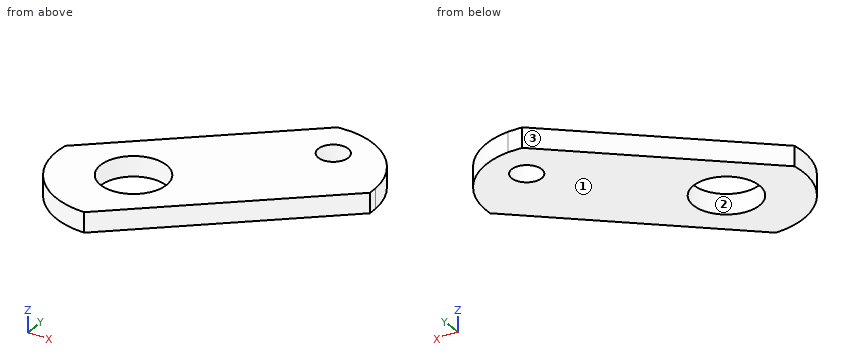
```python
from build123d import *

# Parameters (mm, degrees)
SKETCH1_W           = 38.1
SKETCH1_H           = 30.48
BOSS_EXTRUDE1_DEPTH = 2.54
SKETCH2_R           = 1.905
SKETCH2_R_2         = 4.191
CUT_EXTRUDE1_DEPTH  = 49.857875517
CUT_EXTRUDE3_DEPTH  = 2.54
CUT_EXTRUDE4_DEPTH  = 2.54
CUT_EXTRUDE5_DEPTH  = 2.54


with BuildPart() as part:
    # Sketch1 → Boss-Extrude1 (new body)
    with BuildSketch(Plane.XY):
        with Locations((-19.05, -15.24)):
            Rectangle(SKETCH1_W, SKETCH1_H)
    extrude(amount=BOSS_EXTRUDE1_DEPTH)

    # Sketch2 → Cut-Extrude1 (cut, through all)
    with BuildSketch(Plane.XY.offset(2.54)):
        with Locations((-8.001, -5.08)):
            Circle(SKETCH2_R)
        with Locations((-23.626645651, -20.705645651)):
            Circle(SKETCH2_R_2)
    extrude(amount=-CUT_EXTRUDE1_DEPTH, mode=Mode.SUBTRACT)

    # Sketch3 → Cut-Extrude3 (cut)
    with BuildSketch(Plane.XY.offset(2.54)):
        Polygon((0, -10.322504019), (-23.72616594, -30.48), (0, -30.48), align=None)
        Polygon((-38.1, 0), (-10.660565369, 0), (-38.1, -23.312249215), align=None)
    extrude(amount=-CUT_EXTRUDE3_DEPTH, mode=Mode.SUBTRACT)

    # Sketch4 → Cut-Extrude4 (cut)
    with BuildSketch(Plane.XY.offset(2.54)):
        with BuildLine():
            Line((-38.1, -23.312249215), (-38.1, -30.48))
            Line((-38.1, -30.48), (-23.72616594, -30.48))
            ThreePointArc((-23.72616594, -30.479999994), (-31.076006206, -27.034542439), (-33.288651039, -19.224578768))
            Line((-33.288651039, -19.224578768), (-38.1, -23.312249215))
        make_face()
    extrude(amount=-CUT_EXTRUDE4_DEPTH, mode=Mode.SUBTRACT)

    # Sketch5 → Cut-Extrude5 (cut)
    with BuildSketch(Plane.XY.offset(2.54)):
        with BuildLine():
            Line((0, 0), (-8.85357425, 0))
            ThreePointArc((-8.85357425, 0), (-2.73475248, -2.933386248), (0, -9.143528244))
            Line((0, -9.143528244), (0, 0))
        make_face()
    extrude(amount=-CUT_EXTRUDE5_DEPTH, mode=Mode.SUBTRACT)


solid = part.part
```
Build history of the part. All positions in model axes, mm. Face numbers are marked on the shaded views. Round coordinates to 2 decimals unless told otherwise and drop trailing zeros. Loops run counter-clockwise (first coordinate to the right, second up) from the corner with the lowest first, then second, coordinate; pieces in that order, holes last.
Item 1: Saw through at D-D (x = -19). List the corners of the cut face in (y, z), then the cut area to 3 significant figures.
Item 2: Saw through at C-C (z = 1.45). List the corners of the cut face in (x, y) (1 decimal), then the cut area to 3 significant figures.
Item 3: Two-plate mould, pull along X, no slides. Class the marked faces 1, 2 and 3: released by +X, released by -X, zero draft, split by the parting line, or undercut.
Item 4: Saw through at A-A (y = -5.08). List the corners of the cut face in (x, z).
Item 5: Saw through at B-B (x = -26.5). List the corners of the cut face in (y, z).
Item 6: Drill centre lines: line 1 along Y through (x, z) = (-24, 1.35); line 2 along Y through (x, z) = (-26, 1.05); line 3 along X through (y, z) = (-23, 0.1). Where is each one in solid material? Low to high.
Item 7: Pin check, flat tips, straight feed: P1, Ø3, axis at x = -8.001, y = -5.08, coming from the -Z side; P2, Ø1, axis at x = -23, z = 1.5, coming from the -Y side. Stop position of each tip, or through.
Worked answers:
1. outline: (-26.46, 0) - (-7.09, 0) - (-7.09, 2.54) - (-26.46, 2.54) - close
1. area: 49.2 mm2
2. outline: (-33.3, -19.2) arc R9.8 ccw to (-23.7, -30.5) - (0, -10.3) - (0, -9.1) arc R9.8 ccw to (-8.9, 0) - (-10.7, 0) - close; hole circle Ø8.4 at (-23.6, -20.7); hole circle Ø3.8 at (-8, -5.1)
2. area: 452 mm2
3. face 1: zero draft
3. face 2: undercut
3. face 3: released by -X
4. outline: (-16.64, 0) - (-9.91, 0) - (-9.91, 2.54) - (-16.64, 2.54) - close; (-6.1, 0) - (-1.16, 0) - (-1.16, 2.54) - (-6.1, 2.54) - close
5. outline: (-30.05, 0) - (-23.76, 0) - (-23.76, 2.54) - (-30.05, 2.54) - close; (-17.65, 0) - (-13.46, 0) - (-13.46, 2.54) - (-17.65, 2.54) - close
6. line 1: y = -30.47 to -24.88, -16.53 to -11.33
6. line 2: y = -30.19 to -24.16, -17.25 to -13.03
6. line 3: x = -33.13 to -27.13, -20.12 to -14.92
7. P1: passes through
7. P2: stops at y = -30.29
